Autodesk Inventor part; units mm, degrees
ref_plane "YZ Plane" through (0, 0, 0) normal (1, 0, 0) x (0, 1, 0)
ref_plane "XZ Plane" through (0, 0, 0) normal (0, 1, 0) x (-1, 0, 0)
ref_plane "XY Plane" through (0, 0, 0) normal (0, 0, 1) x (1, 0, 0)
sketch "Náčrt2" plane through (0, 0, 0) normal (1, 0, 0) x (0, 1, 0)
  circle A0 centre (0, 0) radius 6.5
  line L0 (31.5, 12.5) -> (0, 12.5)
  line L1 (31.5, 12.5) -> (31.5, 4.5)
  line L2 (31.5, 4.5) -> (6.4868, -10.6851)
  arc A1 (0, 12.5) -> (6.4868, -10.6851) centre (0, 0) ccw
  dimension "d0" = 13
  dimension "d1" = 6
  dimension "d2" = 31.5
  dimension "d3" = 8
extrude "Vysunutí1" add sketch "Náčrt2" along normal blind 60
fillet "Zaoblení1" radius 4 1 edges at (30, 31.5, 4.5)
chamfer "Zkosení1" distance 0.5 angle 45 2 edges at (0, -6.5, 0) (60, -6.5, 0)
properties part number "DD_KVD_003_10_E" material "Nerezová ocel"
Verification items for the finished model (mm, model axes). Coordinates: 2 decimals unless noted, no trailing zeros. Order: outer loops, then holes, each group sorted by start corner. A loop starts at its lowest first (then second) coordinate and runs counter-clockwise, first axis right, second up. Notation, with made-up numbers: M 34,-4.75 L 87,-4.75 A12 ccw 87,3.25 Z; hole C 26,37.25 d10. An arc over 180 degrees is marked long. One line per item, written item: value. Start each with the question number.
Item 1: Sectioned sample at C-C (y = 18). Enter the section's corners in (x, z), then the cut area to 3 significant figures.
Item 2: Sectioned sample at B-B (z = 0). Enter the section's corners in (x, y), then the cut area to 3 significant figures.
Item 3: Gauge pin test, flat ends, axial feed: pin 1 (6 mm diameter, centred on x = 7, y = 11.5, fed in from -Z); pin 2 (1 mm diameter, centred on x = 11, z = 8.5, fed in from -Y); pin 3 (1 mm diameter, centred on x = 50.5, y = -5, fed in from +Z); pin 4 (11.5 mm diameter, centred on y = 0, z = 0, fed in from +X). Record the tip position at first contact, or that the pin passes through.
Item 4: Sectioned sample at D-D (z = -8.75). Enter the section's corners in (x, y), then the cut area to 3 significant figures.
Item 5: Mould release check, pull along Y, two halves, no side actions. Record for faces 1 (the cylindrical face through (29.587, -5.158, 3.955)), 2 (the flat face through (60, 9, 3)), 3 (the flat face through (30, 31.5, 10)): released by +Y, released by -Y, zero draft, split by the parting line, or undercut.
Item 6: Sectioned sample at A-A (x = 54). Enter the section's corners in (y, z).
Item 7: Scan lines: probe 1 along Z at (x, y) = (26, 0); probe 2 along Y at (x, z) = (43, 4.25); probe 3 along Y at (x, z) = (18.5, 1.5). Record each from-to range of solid material in increasing order.
Conclusion:
1. outline: M 0,-3.7 L 60,-3.7 L 60,12.5 L 0,12.5 Z
1. area: 972 mm^2
2. outline: M 0,-12.5 L 60,-12.5 L 60,-7 L 59.5,-6.5 L 0.5,-6.5 L 0,-7 Z; M 0,7 L 0.5,6.5 L 59.5,6.5 L 60,7 L 60,24.09 L 0,24.09 Z
2. area: 1,410 mm^2
3. pin 1: stops at z = -9.46
3. pin 2: stops at y = -9.6
3. pin 3: stops at z = 11.66
3. pin 4: passes through
4. outline: M 0,-8.93 L 60,-8.93 L 60,9.67 L 0,9.67 Z
4. area: 1,120 mm^2
5. face 1: undercut
5. face 2: zero draft
5. face 3: released by +Y
6. outline: M 0,12.5 A12.5 ccw long 6.49,-10.69 L 29.58,3.33 A4 ccw 31.5,6.75 L 31.5,12.5 Z; hole C 0,0 d13
7. probe 1: z = -12.5 to -6.5, 6.5 to 12.5
7. probe 2: y = -11.76 to -4.92, 4.92 to 30.62
7. probe 3: y = -12.41 to -6.32, 6.32 to 26.56
